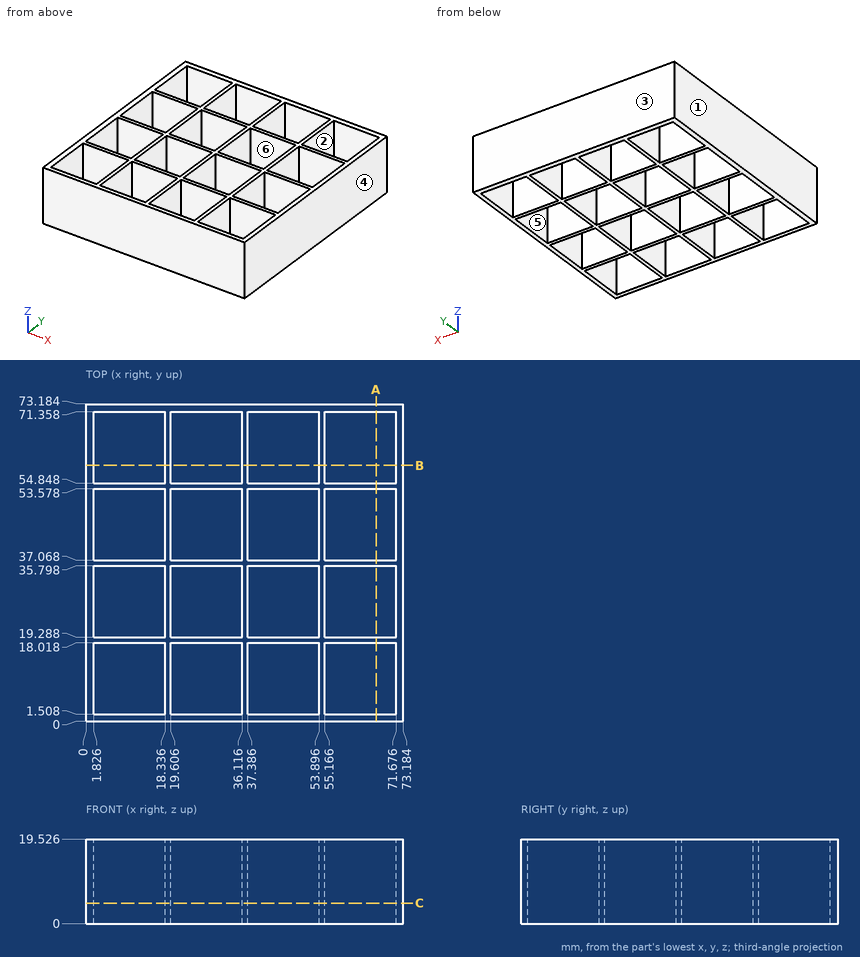
The figure shows three views and two pictorial views of one solid part (mm, origin at its lowest corner). Answer the questions. A direction names the side the tool comes from. Give positions to 0.01 mm unless a question says otherwise; leave off trailing zeros. Write each loop counter-clockwise with the first axis right and the second up, starting at its lowest first coordinate (ties: lowest second). Pieces come first, ordered by that corner, then holes. Notation, with made-up numbers: (52.25, 37.5) -> (63.25, 37.5) arc R19 ccw to (63.25, 74.5) -> close; hole circle Ø4 at (81.5, 88). An arc over 180 degrees is marked (long way). Write each question's results on one line, items separated by ' | '.
1. Determine the mould class of the marked faces 3, 4, 5 and 6 for opening direction X: +X half, -X half, draft (parallel to the pull), parting line (faces both ways), or undercut.
Data:
face 3: draft | face 4: +X half | face 5: undercut | face 6: undercut
2. Find section B-B on y = 59. Determine the outline of the cut face in (x, z) (1 decimal).
Data:
outline: (0, 0) -> (1.8, 0) -> (1.8, 19.5) -> (0, 19.5) -> close; (18.3, 0) -> (19.6, 0) -> (19.6, 19.5) -> (18.3, 19.5) -> close; (36.1, 0) -> (37.4, 0) -> (37.4, 19.5) -> (36.1, 19.5) -> close; (53.9, 0) -> (55.2, 0) -> (55.2, 19.5) -> (53.9, 19.5) -> close; (71.7, 0) -> (73.2, 0) -> (73.2, 19.5) -> (71.7, 19.5) -> close
3. A tool of negligible diameter and unlimited length cuts with its end or side. For the marked faces 1 and 2, from which of +Z, -Z, +X, -X, +Y, -Y can it reach the whole face along a straight path? Write none if from no direction.
Data:
face 1: +Z, -Z, -X, +Y, -Y | face 2: +Z, -Z
4. Straight lines are drawn through the part: L1, parallel to X at y = 45, z = 18.5 (1 decimal); L2, parallel to Y at x = 45.5, z = 17.25. For each, find the intervals that lie inside material, in ascending order.
Data:
L1: 0 to 1.8, 18.3 to 19.6, 36.1 to 37.4, 53.9 to 55.2, 71.7 to 73.2 | L2: 0 to 1.51, 18.02 to 19.29, 35.8 to 37.07, 53.58 to 54.85, 71.36 to 73.18
5. Find section A-A on x = 67. Determine the outline of the cut face in (y, z).
Data:
outline: (0, 0) -> (1.51, 0) -> (1.51, 19.53) -> (0, 19.53) -> close; (18.02, 0) -> (19.29, 0) -> (19.29, 19.53) -> (18.02, 19.53) -> close; (35.8, 0) -> (37.07, 0) -> (37.07, 19.53) -> (35.8, 19.53) -> close; (53.58, 0) -> (54.85, 0) -> (54.85, 19.53) -> (53.58, 19.53) -> close; (71.36, 0) -> (73.18, 0) -> (73.18, 19.53) -> (71.36, 19.53) -> close
6. Find section C-C on z = 4.75. Give the number of separate pieces and of enclosed holes in the cut face.
Data:
separate pieces: 1 | enclosed holes: 16
